The listing builds one solid part. Answer for the finished solid, in the listing's coordinates (mm). Coordinates: 2 decimals unless noted, no trailing zeros. Write each loop counter-clockwise with the first axis right and the second up, starting at its lowest first coordinate (ties: lowest second). Pieces come first, ordered by that corner, then holes.
from build123d import *

# Parameters (mm, degrees)
BOSS_EXTRUDE2_DEPTH = 0.25


with BuildPart() as part:
    # Sketch1 → Boss-Extrude2 (new body)
    with BuildSketch(Plane(origin=(0, 0, 0), x_dir=(-1, 0, 0), z_dir=(0, 0, 1))):
        with BuildLine():
            ThreePointArc((27, 8.310385069), (0, 28.25), (-27, 8.310385069))
            Line((-27, 8.310385069), (-27, -8.310385069))
            ThreePointArc((-27, -8.310385069), (0, -28.25), (27, -8.310385069))
            Line((27, -8.310385069), (27, 8.310385069))
        make_face()
        with BuildLine():
            Line((18.384776311, 16.970562748), (17.485999772, 16.07178621))
            ThreePointArc((17.485999772, 16.07178621), (22.128657829, 8.624674064), (23.75, 0))
            ThreePointArc((23.75, 0), (22.128657829, -8.624674064), (17.485999772, -16.07178621))
            Line((17.485999772, -16.07178621), (18.384776311, -16.970562748))
            ThreePointArc((18.384776311, -16.970562748), (18.384776311, -18.384776311), (16.970562748, -18.384776311))
            Line((16.970562748, -18.384776311), (16.07178621, -17.485999772))
            ThreePointArc((16.07178621, -17.485999772), (0, -23.75), (-16.07178621, -17.485999772))
            Line((-16.07178621, -17.485999772), (-16.970562748, -18.384776311))
            ThreePointArc((-16.970562748, -18.384776311), (-18.384776311, -18.384776311), (-18.384776311, -16.970562748))
            Line((-18.384776311, -16.970562748), (-17.485999772, -16.07178621))
            ThreePointArc((-17.485999772, -16.07178621), (-23.75, 0), (-17.485999772, 16.07178621))
            Line((-17.485999772, 16.07178621), (-18.384776311, 16.970562748))
            ThreePointArc((-18.384776311, 16.970562748), (-18.384776311, 18.384776311), (-16.970562748, 18.384776311))
            Line((-16.970562748, 18.384776311), (-16.07178621, 17.485999772))
            ThreePointArc((-16.07178621, 17.485999772), (0, 23.75), (16.07178621, 17.485999772))
            Line((16.07178621, 17.485999772), (16.970562748, 18.384776311))
            ThreePointArc((16.970562748, 18.384776311), (18.384776311, 18.384776311), (18.384776311, 16.970562748))
        make_face(mode=Mode.SUBTRACT)
    extrude(amount=BOSS_EXTRUDE2_DEPTH)


solid = part.part
1. Find the intervals of material crossed by L1, parallel to X at y = -0.5, z = 0.1; L2, parallel to Y at x = 18, z = 0.1; L3, parallel to Y at x = 2, z = 0.15, in increasing order.
Results found:
L1: x = -27 to -23.74, 23.74 to 27
L2: y = -21.77 to -18.62, -16.59 to -15.49, 15.49 to 16.59, 18.62 to 21.77
L3: y = -28.18 to -23.67, 23.67 to 28.18
2. Section A-A on x = 0 is taken. Give the vertices of the cut face in (y, z), then the cut area to 3 significant figures.
Results found:
outline: (-28.25, 0) - (-23.75, 0) - (-23.75, 0.25) - (-28.25, 0.25) - close; (23.75, 0) - (28.25, 0) - (28.25, 0.25) - (23.75, 0.25) - close
area: 2.25 mm2
3. A flat-ended cylindrical pin translates along its axis: P1, Ø1, axis at x = 15, y = -16, coming from the +Z side (3 decimals). Find the tip coordinate at first contact, or state that the pin passes through.
Results found:
P1: passes through
4. Section D-D on y = 24.5 is taken. Give the vertices of the cut face in (x, z), then the cut area to 3 significant figures.
Results found:
outline: (-14.06, 0) - (14.06, 0) - (14.06, 0.25) - (-14.06, 0.25) - close
area: 7.03 mm2
5. Section C-C on y = -22 is taken. Give the vertices of the cut face in (x, z), then the cut area to 3 significant figures.
Results found:
outline: (-17.72, 0) - (-8.95, 0) - (-8.95, 0.25) - (-17.72, 0.25) - close; (8.95, 0) - (17.72, 0) - (17.72, 0.25) - (8.95, 0.25) - close
area: 4.39 mm2
6. Section B-B on z = 0.1 is taken. Give the vertices of the cut face in (x, y).
Results found:
outline: (-27, -8.31) arc R28.25 ccw to (27, -8.31) - (27, 8.31) arc R28.25 ccw to (-27, 8.31) - close; hole (-18.38, -16.97) arc R1 ccw to (-16.97, -18.38) - (-16.07, -17.49) arc R23.75 ccw to (16.07, -17.49) - (16.97, -18.38) arc R1 ccw to (18.38, -16.97) - (17.49, -16.07) arc R23.75 ccw to (17.49, 16.07) - (18.38, 16.97) arc R1 ccw to (16.97, 18.38) - (16.07, 17.49) arc R23.75 ccw to (-16.07, 17.49) - (-16.97, 18.38) arc R1 ccw to (-18.38, 16.97) - (-17.49, 16.07) arc R23.75 ccw to (-17.49, -16.07) - close
